The listing builds one solid part. Answer for the finished solid, in the listing's coordinates (mm). A direction names the side the tool comes from. Round coordinates to 2 decimals unless told otherwise and drop trailing zeros. Write each loop counter-clockwise with the first axis right and the second up, starting at its lowest first coordinate (ties: lowest second). Pieces come first, ordered by that corner, then holes.
(1) A cutting plane is placed at D-D, the plane z = 3.05. Give the number of separate pieces and of enclosed holes in the cut face, and give its area (3 significant figures).
(2) Each of these flat-tipped pins is pushed along its axis until it touches: pin 1 Ø1.1 at (y, z) = (2, 5.5) entering from -X; pin 2 Ø1 at (x, z) = (-3, 5) entering from +Y; pin 3 Ø4 at (x, z) = (0.5, 5.5) entering from -Y. Where does it stop, or does it pass through?
(3) Find the intervals of material crossed by probe 1 along X at (y, z) = (1.7, 7); probe 2 along X at (y, z) = (0.9, 0.75); probe 3 along Y at (x, z) = (0.75, 4), in increasing order.
(4) The mould has two halves that part along Y. Classify faces 6 (the face through (1.05, 2, 5)), 7 (the face through (-3, 1, 0)), 8 (the face through (0, 0, 4)): +Y half, -Y half, draft (parallel to the pull), parting line (faces both ways), or undercut.
(5) A cutting plane is placed at B-B, the plane x = 2.75. Give the vertices of the cut face in (y, z).
(6) A cutting plane is placed at A-A, the plane z = 7.25. Give the vertices of the cut face in (x, y), and give its area (3 significant figures).
(7) For faces 1 (the face through (-2.015, -0.444, 2.695)), 2 (the face through (0, 3.1, 2)), 3 (the face through (1.85, 0.9, 0.5)), 4 (the face through (-3.55, 1, 2)), 5 (the face through (0, 0.3, 4.8)), determine the directions among +Z, -Z, +X, -X, +Y, -Y from which every point of the face is accessible in a straight line to the end or side of a thin tool.
(8) A cutting plane is placed at C-C, the plane y = -0.4. Give the vertices of the cut face in (x, z), and give its area (3 significant figures).
from build123d import *

# Parameters (mm, degrees)
BOSS_EXTRUDE1_DEPTH = 8.2
BOSS_EXTRUDE2_DEPTH = 3.85
SKETCH3_OUTSIDE_W   = 12.05
SKETCH3_OUTSIDE_H   = 7.75
CUT_EXTRUDE1_DEPTH  = 4.8
SKETCH4_W           = 1
SKETCH4_H           = 0.3
CUT_EXTRUDE3_DEPTH  = 2.3
CUT_EXTRUDE6_DEPTH  = 4.4
SKETCH6_W           = 0.5
SKETCH6_H           = 0.5
CUT_EXTRUDE7_DEPTH  = 2
SKETCH7_W           = 0.5
SKETCH7_H           = 0.8
CUT_EXTRUDE8_DEPTH  = 7
SKETCH8_W           = 6
SKETCH8_H           = 1
CUT_EXTRUDE9_DEPTH  = 2
SKETCH9_W           = 6
SKETCH9_H           = 0.5
CUT_EXTRUDE10_DEPTH = 1
SKETCH10_R          = 0.4
BOSS_EXTRUDE3_DEPTH = 1.1
CHAMFER1_SIZE       = 0.2
SKETCH11_W          = 7.1
SKETCH11_H          = 0.3
BOSS_EXTRUDE4_DEPTH = 3.7
FILLET1_R           = 0.2
SKETCH12_W          = 3
SKETCH12_H          = 2
CUT_EXTRUDE11_DEPTH = 0.5
FILLET2_R           = 0.2
FILLET3_R           = 0.4


with BuildPart() as part:
    # Sketch1 → Boss-Extrude1 (new body)
    with BuildSketch(Plane.XY):
        with BuildLine():
            Line((-3.25, 3.4), (3.25, 3.4))
            ThreePointArc((3.25, 3.4), (3.462132034, 3.312132034), (3.55, 3.1))
            Line((3.55, 3.1), (3.55, 0))
            Line((3.55, 0), (-3.55, 0))
            Line((-3.55, 0), (-3.55, 3.1))
            ThreePointArc((-3.55, 3.1), (-3.462132034, 3.312132034), (-3.25, 3.4))
        make_face()
    extrude(amount=BOSS_EXTRUDE1_DEPTH)

    # Sketch2 → Boss-Extrude2 (add, symmetric)
    with BuildSketch(Plane(origin=(0, 0, 0), x_dir=(0, 0, -1), z_dir=(1, 0, 0))):
        with BuildLine():
            Line((0, 2.25), (-3.3, 2.25))
            ThreePointArc((-3.3, 2.25), (-3.7, 1.85), (-3.3, 1.45))
            Line((-3.3, 1.45), (0, 1.45))
            Line((0, 1.45), (0, 2.25))
        make_face()
    extrude(amount=BOSS_EXTRUDE2_DEPTH, both=True)

    # Sketch3 outside → Cut-Extrude1 (cut)
    with BuildSketch(Plane.XY.offset(8.2)):
        with Locations((0, 1.7)):
            Rectangle(SKETCH3_OUTSIDE_W, SKETCH3_OUTSIDE_H)
        with BuildLine():
            Line((-2, 2.2), (2, 2.2))
            ThreePointArc((2, 2.2), (2.212132034, 2.112132034), (2.3, 1.9))
            Line((2.3, 1.9), (2.3, 1.1))
            Line((2.3, 1.1), (1.8, 0.6))
            Line((1.8, 0.6), (-1.8, 0.6))
            Line((-1.8, 0.6), (-2.3, 1.1))
            Line((-2.3, 1.1), (-2.3, 1.9))
            ThreePointArc((-2.3, 1.9), (-2.212132034, 2.112132034), (-2, 2.2))
        make_face(mode=Mode.SUBTRACT)
    extrude(amount=-CUT_EXTRUDE1_DEPTH, mode=Mode.SUBTRACT)

    # Sketch4 → Cut-Extrude3 (cut)
    with BuildSketch(Plane.XY):
        with Locations((0, 3.25)):
            Rectangle(SKETCH4_W, SKETCH4_H)
    extrude(amount=CUT_EXTRUDE3_DEPTH, mode=Mode.SUBTRACT)

    # Sketch5 → Cut-Extrude6 (cut, through all)
    with BuildSketch(Plane(origin=(0, 0, 0), x_dir=(1, 0, 0), z_dir=(0, 1, 0))):
        Polygon((-1.85, 0), (1.85, 0), (1.85, -1), (1.35, -1), (1.35, -0.7), (1.05, -0.7), (1.05, -1), (0.55, -1), (0.55, -0.7), (0.25, -0.7), (0.25, -1), (-0.25, -1), (-0.25, -0.7), (-0.55, -0.7), (-0.55, -1), (-1.05, -1), (-1.05, -0.7), (-1.35, -0.7), (-1.35, -1), (-1.85, -1), align=None)
    extrude(amount=CUT_EXTRUDE6_DEPTH, mode=Mode.SUBTRACT)

    # Sketch6 → Cut-Extrude7 (cut)
    with BuildSketch(Plane.XY.offset(8.2)):
        with Locations((1.6, 1.65)):
            Rectangle(SKETCH6_W, SKETCH6_H)
        with Locations((0.8, 1.65)):
            Rectangle(SKETCH6_W, SKETCH6_H)
        with Locations((0, 1.65)):
            Rectangle(SKETCH6_W, SKETCH6_H)
        with Locations((-0.8, 1.65)):
            Rectangle(SKETCH6_W, SKETCH6_H)
        with Locations((-1.6, 1.65)):
            Rectangle(SKETCH6_W, SKETCH6_H)
    extrude(amount=-CUT_EXTRUDE7_DEPTH, mode=Mode.SUBTRACT)

    # Sketch7 → Cut-Extrude8 (cut)
    with BuildSketch(Plane.XY):
        with Locations((1.6, 2)):
            Rectangle(SKETCH7_W, SKETCH7_H)
        with Locations((0.8, 2)):
            Rectangle(SKETCH7_W, SKETCH7_H)
        with Locations((0, 2)):
            Rectangle(SKETCH7_W, SKETCH7_H)
        with Locations((-0.8, 2)):
            Rectangle(SKETCH7_W, SKETCH7_H)
        with Locations((-1.6, 2)):
            Rectangle(SKETCH7_W, SKETCH7_H)
    extrude(amount=CUT_EXTRUDE8_DEPTH, mode=Mode.SUBTRACT)

    # Sketch8 → Cut-Extrude9 (cut)
    with BuildSketch(Plane(origin=(0, 3.4, 0), x_dir=(1, 0, 0), z_dir=(0, 1, 0))):
        with Locations((0, -0.5)):
            Rectangle(SKETCH8_W, SKETCH8_H)
    extrude(amount=-CUT_EXTRUDE9_DEPTH, mode=Mode.SUBTRACT)

    # Sketch9 → Cut-Extrude10 (cut)
    with BuildSketch(Plane.XY):
        with Locations((0, 0.25)):
            Rectangle(SKETCH9_W, SKETCH9_H)
    extrude(amount=CUT_EXTRUDE10_DEPTH, mode=Mode.SUBTRACT)

    # Sketch10 → Boss-Extrude3 (add)
    with BuildSketch(Plane.XZ):
        with Locations((2.2, 3.05)):
            Circle(SKETCH10_R)
        with Locations((-2.2, 3.05)):
            Circle(SKETCH10_R)
    extrude(amount=BOSS_EXTRUDE3_DEPTH)

    # Chamfer1
    chamfer1_edges = [part.edges().sort_by_distance(p)[0] for p in [
        (1.8, -1.1, 3.05),
        (-2.6, -1.1, 3.05),
    ]]
    chamfer(chamfer1_edges, length=CHAMFER1_SIZE)

    # Sketch11 → Boss-Extrude4 (add)
    with BuildSketch(Plane.XY.offset(3.4)):
        with Locations((0, 0.15)):
            Rectangle(SKETCH11_W, SKETCH11_H)
    extrude(amount=BOSS_EXTRUDE4_DEPTH)

    # Fillet1
    fillet1_edges = [part.edges().sort_by_distance(p)[0] for p in [
        (-3.55, 0.15, 7.1),
        (3.55, 0.15, 7.1),
    ]]
    fillet(fillet1_edges, radius=FILLET1_R)

    # Sketch12 → Cut-Extrude11 (cut)
    with BuildSketch(Plane.XZ):
        with Locations((0, 6.1)):
            Rectangle(SKETCH12_W, SKETCH12_H)
    extrude(amount=-CUT_EXTRUDE11_DEPTH, mode=Mode.SUBTRACT)

    # Fillet2
    fillet2_edges = [part.edges().sort_by_distance(p)[0] for p in [
        (1.5, 0.15, 5.1),
        (-1.5, 0.15, 5.1),
    ]]
    fillet(fillet2_edges, radius=FILLET2_R)

    # Fillet3
    fillet3_edges = [part.edges().sort_by_distance(p)[0] for p in [
        (1.5, 0.15, 7.1),
        (-1.5, 0.15, 7.1),
    ]]
    fillet(fillet3_edges, radius=FILLET3_R)


solid = part.part
Solutions:
1. separate pieces: 1
1. enclosed holes: 5
1. area: 24.3 mm2
2. pin 1: stops at x = -2.3
2. pin 2: stops at y = 0.3
2. pin 3: stops at y = 0
3. probe 1: x = -2.3 to -1.85, -1.35 to -1.05, -0.55 to -0.25, 0.25 to 0.55, 1.05 to 1.35, 1.85 to 2.3
3. probe 2: x = -3.55 to -1.85, -1.35 to -1.05, -0.55 to -0.25, 0.25 to 0.55, 1.05 to 1.35, 1.85 to 3.55
3. probe 3: y = 0 to 0.3, 0.6 to 1.6
4. face 6: undercut
4. face 7: draft
4. face 8: -Y half
5. outline: (0, 1) - (0.5, 1) - (0.5, 0) - (1.4, 0) - (1.4, 1) - (3.4, 1) - (3.4, 3.4) - (0.3, 3.4) - (0.3, 7.1) - (0, 7.1) - close
6. outline: (-2.3, 1.1) - (-1.8, 0.6) - (1.8, 0.6) - (2.3, 1.1) - (2.3, 1.9) arc R0.3 ccw to (2, 2.2) - (-2, 2.2) arc R0.3 ccw to (-2.3, 1.9) - close; hole (-1.85, 1.4) - (-1.35, 1.4) - (-1.35, 1.9) - (-1.85, 1.9) - close; hole (-1.05, 1.4) - (-0.55, 1.4) - (-0.55, 1.9) - (-1.05, 1.9) - close; hole (-0.25, 1.4) - (0.25, 1.4) - (0.25, 1.9) - (-0.25, 1.9) - close; hole (0.55, 1.4) - (1.05, 1.4) - (1.05, 1.9) - (0.55, 1.9) - close; hole (1.35, 1.4) - (1.85, 1.4) - (1.85, 1.9) - (1.35, 1.9) - close
6. area: 5.82 mm2
7. face 1: -Y
7. face 2: -Z, +Y
7. face 3: -Z, +Y, -Y
7. face 4: +Z, -Z, -X, -Y
7. face 5: +Z, +X, -X
8. outline: circle Ø0.8 at (-2.2, 3.05); circle Ø0.8 at (2.2, 3.05)
8. area: 1.01 mm2
